```python
from build123d import *

# Parameters (mm, degrees)
BOSS_EXTRUDE1_DEPTH                             = 130
BOSS_EXTRUDE1_DEPTH_BACK                        = 16
SKETCH1_W                                       = 55
SKETCH1_H                                       = 55
SKETCH1_W_2                                     = 45
SKETCH1_H_2                                     = 42
SKETCH2_W                                       = 40
SKETCH2_H                                       = 35
CUT_EXTRUDE1_DEPTH                              = 168
CUT_EXTRUDE2_DEPTH                              = 10
SKETCH8_W                                       = 25
SKETCH8_H                                       = 8
CUT_EXTRUDE5_DEPTH                              = 5
CSK_FOR_M2_FLAT_HEAD_MACHINE_SCREW2_D           = 2.4
CSK_FOR_M2_FLAT_HEAD_MACHINE_SCREW2_DEPTH       = 9.278967257
CSK_FOR_M2_FLAT_HEAD_MACHINE_SCREW2_CSINK_D     = 4.4
CSK_FOR_M2_FLAT_HEAD_MACHINE_SCREW2_CSINK_ANGLE = 90
CSK_FOR_M2_FLAT_HEAD_MACHINE_SCREW2_TIP         = 0.721032743
CHAMFER1_SIZE                                   = 1
CHAMFER3_SIZE                                   = 1
CUT_EXTRUDE6_REACH                              = 153.131
SKETCH11_W                                      = 20
SKETCH11_H                                      = 10
CUT_EXTRUDE7_REACH                              = 145.81
SKETCH12_R                                      = 1.7
CHAMFER2_SIZE                                   = 5
SKETCH13_R                                      = 1.2
CUT_EXTRUDE8_DEPTH                              = 10


with BuildPart() as part:
    # Sketch1 → Boss-Extrude1 (new, two sides: drawn at the far end of the back side and taken through both)
    with BuildSketch(Plane(origin=(0, 0, 0), x_dir=(1, 0, 0), z_dir=(0, 1, 0)).offset(-BOSS_EXTRUDE1_DEPTH_BACK)):
        Rectangle(SKETCH1_W, SKETCH1_H)
        with Locations((0, -1.5)):
            Rectangle(SKETCH1_W_2, SKETCH1_H_2, mode=Mode.SUBTRACT)
    extrude(amount=BOSS_EXTRUDE1_DEPTH + BOSS_EXTRUDE1_DEPTH_BACK)

    # Sketch2 → Cut-Extrude1 (cut)
    with BuildSketch(Plane.XY.offset(27.5)):
        with Locations((0, 17.5)):
            Rectangle(SKETCH2_W, SKETCH2_H)
    extrude(amount=-CUT_EXTRUDE1_DEPTH, mode=Mode.SUBTRACT)

    # Sketch7 → Cut-Extrude2 (cut)
    with BuildSketch(Plane(origin=(0, 0, -27.5), x_dir=(-1, 0, 0), z_dir=(0, 0, -1))):
        Polygon((19.5, 41.7), (22.5, 44.7), (22.5, 78.7), (19.5, 81.7), (-19.5, 81.7), (-22.5, 78.7), (-22.5, 44.7), (-19.5, 41.7), align=None)
    extrude(amount=-CUT_EXTRUDE2_DEPTH, mode=Mode.SUBTRACT)

    # Sketch8 → Cut-Extrude5 (cut)
    with BuildSketch(Plane.XZ.offset(-81.7)):
        with Locations((0, -23.5)):
            Rectangle(SKETCH8_W, SKETCH8_H)
    extrude(amount=-CUT_EXTRUDE5_DEPTH, mode=Mode.SUBTRACT)

    # CSK for M2 Flat Head Machine Screw2
    with Locations(Plane(origin=(0, 86.7, 0), x_dir=(-1, 0, 0), z_dir=(0, -1, 0))):
        with Locations((-5.5, 23.5), (5.5, 23.5)):
            CounterSinkHole(CSK_FOR_M2_FLAT_HEAD_MACHINE_SCREW2_D / 2, CSK_FOR_M2_FLAT_HEAD_MACHINE_SCREW2_CSINK_D / 2, depth=CSK_FOR_M2_FLAT_HEAD_MACHINE_SCREW2_DEPTH, counter_sink_angle=CSK_FOR_M2_FLAT_HEAD_MACHINE_SCREW2_CSINK_ANGLE)
            with Locations((0, 0, -(CSK_FOR_M2_FLAT_HEAD_MACHINE_SCREW2_DEPTH + CSK_FOR_M2_FLAT_HEAD_MACHINE_SCREW2_TIP / 2))):  # 118° drill point
                Cone(0, CSK_FOR_M2_FLAT_HEAD_MACHINE_SCREW2_D / 2, CSK_FOR_M2_FLAT_HEAD_MACHINE_SCREW2_TIP, mode=Mode.SUBTRACT)

    # Chamfer1
    chamfer1_edges = [part.edges().sort_by_distance(p)[0] for p in [
        (-22.5, 57, 22.5),
        (22.5, 57, 22.5),
        (22.5, 14.35, -19.5),
        (-22.5, 14.35, -19.5),
        (22.5, 104.35, -19.5),
        (-22.5, 104.35, -19.5),
    ]]
    chamfer(chamfer1_edges, length=CHAMFER1_SIZE)

    # Chamfer3
    chamfer3_edges = [part.edges().sort_by_distance(p)[0] for p in [
        (27.5, 57, 27.5),
        (-27.5, 57, 27.5),
        (-27.5, 57, -27.5),
        (27.5, 57, -27.5),
    ]]
    chamfer(chamfer3_edges, length=CHAMFER3_SIZE)

    # Sketch11 → Cut-Extrude6 (cut, up to next)
    with BuildSketch(Plane(origin=(-27, 0, 27), x_dir=(0.7071067811865475, 0, 0.7071067811865477), z_dir=(-0.7071067811865477, 0, 0.7071067811865475)), mode=Mode.PRIVATE) as cut_extrude6_sk1:
        with Locations((0, 125)):
            Rectangle(SKETCH11_W, SKETCH11_H)
    cut_extrude6_tool1 = extrude(cut_extrude6_sk1.sketch, amount=-CUT_EXTRUDE6_REACH, mode=Mode.PRIVATE) & part.part
    add(cut_extrude6_tool1.solids().sort_by_distance((-27, 125, 27))[0], mode=Mode.SUBTRACT)

    # Sketch12 → Cut-Extrude7 (cut, up to next)
    with BuildSketch(Plane(origin=(27.5, 0, 0), x_dir=(0, 0, -1), z_dir=(1, 0, 0)), mode=Mode.PRIVATE) as cut_extrude7_sk1:
        with Locations((9.5, 7)):
            Circle(SKETCH12_R)
    cut_extrude7_tool1 = extrude(cut_extrude7_sk1.sketch, amount=-CUT_EXTRUDE7_REACH, mode=Mode.PRIVATE) & part.part
    # Sketch12 → Cut-Extrude7 (cut, up to next)
    with BuildSketch(Plane(origin=(27.5, 0, 0), x_dir=(0, 0, -1), z_dir=(1, 0, 0)), mode=Mode.PRIVATE) as cut_extrude7_sk2:
        with Locations((-15.5, 7)):
            Circle(SKETCH12_R)
    cut_extrude7_tool2 = extrude(cut_extrude7_sk2.sketch, amount=-CUT_EXTRUDE7_REACH, mode=Mode.PRIVATE) & part.part
    # Sketch12 → Cut-Extrude7 (cut, up to next)
    with BuildSketch(Plane(origin=(27.5, 0, 0), x_dir=(0, 0, -1), z_dir=(1, 0, 0)), mode=Mode.PRIVATE) as cut_extrude7_sk3:
        with Locations((-15.5, 23)):
            Circle(SKETCH12_R)
    cut_extrude7_tool3 = extrude(cut_extrude7_sk3.sketch, amount=-CUT_EXTRUDE7_REACH, mode=Mode.PRIVATE) & part.part
    # Sketch12 → Cut-Extrude7 (cut, up to next)
    with BuildSketch(Plane(origin=(27.5, 0, 0), x_dir=(0, 0, -1), z_dir=(1, 0, 0)), mode=Mode.PRIVATE) as cut_extrude7_sk4:
        with Locations((9.5, 23)):
            Circle(SKETCH12_R)
    cut_extrude7_tool4 = extrude(cut_extrude7_sk4.sketch, amount=-CUT_EXTRUDE7_REACH, mode=Mode.PRIVATE) & part.part
    add(cut_extrude7_tool1.solids().sort_by_distance((27.5, 7, -9.5))[0], mode=Mode.SUBTRACT)
    add(cut_extrude7_tool2.solids().sort_by_distance((27.5, 7, 15.5))[0], mode=Mode.SUBTRACT)
    add(cut_extrude7_tool3.solids().sort_by_distance((27.5, 23, 15.5))[0], mode=Mode.SUBTRACT)
    add(cut_extrude7_tool4.solids().sort_by_distance((27.5, 23, -9.5))[0], mode=Mode.SUBTRACT)

    # Chamfer2
    chamfer2_edges = [part.edges().sort_by_distance(p)[0] for p in [
        (0, 35, -27.5),
        (0, 0, -27.5),
        (0, 35, 27.5),
        (0, 0, 27.5),
    ]]
    chamfer(chamfer2_edges, length=CHAMFER2_SIZE - 0.0001)  # a hair under: the kernel refuses the full size

    # Sketch13 → Cut-Extrude8 (cut)
    with BuildSketch(Plane(origin=(0, 130, 0), x_dir=(1, 0, 0), z_dir=(0, 1, 0))):
        with Locations(Location((0, 23.5, 0), (0, 0, 270))):
            Circle(SKETCH13_R)
        with Locations(Location((0, -25, 0), (0, 0, 270))):
            Circle(SKETCH13_R)
        with Locations(Location((25, 0, 0), (0, 0, 270))):
            Circle(SKETCH13_R)
        with Locations(Location((-25, 0, 0), (0, 0, 270))):
            Circle(SKETCH13_R)
    extrude(amount=-CUT_EXTRUDE8_DEPTH, mode=Mode.SUBTRACT)


solid = part.part
```
Could you check a few things on this model? Use its own coordinates, in mm. A direction names the side the tool comes from. Round coordinates to 2 decimals unless told otherwise and drop trailing zeros. Order: outer loops, then holes, each group sorted by start corner. A loop starts at its lowest first (then second) coordinate and runs counter-clockwise, first axis right, second up. Notation, with made-up numbers: M 87,-40 L 121,-40 A22 ccw 121,-1 Z; hole C 21.25,14.5 d3. An arc over 180 degrees is marked long. One line per question, with ' | ' between items. Start each with the question number.
(1) For faces 1 (the face through (25.04, 5.34, -9.13)), 2 (the face through (12.5, 84, -24)), 3 (the face through (1, -2, -19.5)), 4 (the face through (-20, 17, 25)), which set-ups out of +Z, -Z, +X, -X, +Y, -Y let a thin tool reach every point of the face, with its end or its side?
(2) Suppose I cut it at C-C on z = -9.5. List the corners of the cut face in (x, y) for me, then the cut area to 3 significant figures.
(3) Suppose I cut it at D-D on y = 100. List the corners of the cut face in (x, z) for me.
(4) Suppose I cut it at A-A on y = 7. Count the separate pieces of the cut face and the enclosed holes in it, then the cut area to 3 significant figures.
(5) For P1, Ø3, axis at x = 20.5, y = 76.5, coming from the -Z side, with a flat end and sliding along its axis, tell me the tip position at first contact or that it passes through.
(6) Thinking about a two-plate mould opening in Z: for faces 5 (the face through (21, 43.2, -23.1)), 6 (the face through (-10.893, 124.93, 25.035)), 7 (the face through (-25.035, 124.93, 10.893)), which applies, +Z half, -Z half, draft (parallel to the pull), parting line (faces both ways), or undercut?
(7) Please list where these lines run through material, in increasing order: line 1 along Y through (x, z) = (23.6, 15.5); line 2 along Z through (x, y) = (5.5, 91.75); line 3 along X through (y, z) = (61.5, 0).
Geometry results:
1) face 1: +X | face 2: -Z | face 3: +Y, -Y | face 4: +Z
2) outline: M -27.5,-16 L -22.5,-16 L -22.5,130 L -27.5,130 Z; M 22.5,-16 L 27.5,-16 L 27.5,5.3 L 22.5,5.3 Z; M 22.5,8.7 L 27.5,8.7 L 27.5,21.3 L 22.5,21.3 Z; M 22.5,24.7 L 27.5,24.7 L 27.5,130 L 22.5,130 Z | area: 1,430 mm²
3) outline: M -27.5,-26.5 L -26.5,-27.5 L 26.5,-27.5 L 27.5,-26.5 L 27.5,26.5 L 26.5,27.5 L -26.5,27.5 L -27.5,26.5 Z; hole M -22.5,-18.5 L -21.5,-19.5 L 21.5,-19.5 L 22.5,-18.5 L 22.5,21.5 L 21.5,22.5 L -21.5,22.5 L -22.5,21.5 Z
4) separate pieces: 4 | enclosed holes: 0 | area: 581 mm²
5) P1: z = 22
6) face 5: draft | face 6: undercut | face 7: +Z half
7) line 1: -16 to 5.3, 8.7 to 21.3, 24.7 to 130 | line 2: -27.5 to -24.7, -22.3 to -19.5, 22.5 to 27.5 | line 3: -27.5 to -22.5, 22.5 to 27.5
